```python
from build123d import *

# Parameters (mm, degrees)
F0_W     = 75
F0_H     = 21.8987613916
F1_DEPTH = 14
F3_DEPTH = 21.8997613916
F4_W     = 23.978275167
F4_H     = 7.947247941
F4_W_2   = 48.6262406095
F5_DEPTH = 25
F6_W     = 7.6308213174
F6_H     = 13.8987613916
F6_W_2   = 6.0403123498
F6_W_3   = 10.3618325666
F7_DEPTH = 6


with BuildPart() as f1:
    # F0 (on Top) → F1 (new body)
    with BuildSketch(Plane.XY):
        with Locations((37.5, 10.9493806958)):
            Rectangle(F0_W, F0_H)
    extrude(amount=F1_DEPTH)

    # F2 (on face) → F3 (cut, through all)
    with BuildSketch(Plane.XZ):
        Polygon((0, 14), (0, 6.3767037354), (5.3324829787, 14), align=None)
        Polygon((68.8854381442, 14), (11.3727953285, 14), (13.736397028, 6.2453923747), (62.3593553901, 6.8103666529), (63.1077513099, 9.8052984104), (65.2087256312, 11.3810319453), (67.0470818877, 12.6941427588), align=None)
        Polygon((75, 14), (70.9864199162, 14), (73.8660361752, 12.6941427588), (75, 10.330542922), align=None)
        Polygon((67.3934295774, 4.770135507), (67.3934295774, 0), (75, 0), (75, 2.5454831775), (74.345, 2.5454831775), (74.345, 4.770135507), align=None)
        Polygon((2.3223445751, 6.9947880693), (0, 4.561574664), (0, 0), (9.3439053744, 2.0588401239), (8.8216059457, 6.9350752235), (8.1620588899, 7.2728698142), (6.6326097585, 4.2866062695), (5.1598150908, 4.2866062695), align=None)
    extrude(amount=-F3_DEPTH, mode=Mode.SUBTRACT)

    # F4 (on face) → F5 (cut)
    with BuildSketch(Plane(origin=(-0.0707041789, 0, 6.0849608152), x_dir=(0.9999325005, 0, 0.0116187119), z_dir=(-0.0116187119, 0, 0.9999325005))):
        with Locations((74.4234114354, 11.0779821407)):
            Rectangle(F4_W, F4_H)
        with Locations((38.1211535471, 11.0779821407)):
            Rectangle(F4_W_2, F4_H)
    extrude(amount=F5_DEPTH, mode=Mode.SUBTRACT)

    # F6 (on face) → F7 (cut)
    with BuildSketch(Plane.XY.offset(14)):
        with Locations((15.1882059872, 10.9493806958)):
            Rectangle(F6_W, F6_H)
        with Locations((8.3526391536, 10.9493806958)):
            Rectangle(F6_W_2, F6_H)
        with Locations((0.1515666954, 10.9493806958)):
            Rectangle(F6_W_3, F6_H)
    extrude(amount=-F7_DEPTH, mode=Mode.SUBTRACT)


solid = f1.part
```
Source: CAD feature listing. Evaluate the final solid. Frame: model axes, mm. A direction names the side the tool comes from. Give positions to 0.01 mm unless a question says otherwise; leave off trailing zeros. Order: outer loops, then holes, each group sorted by start corner. A loop starts at its lowest first (then second) coordinate and runs counter-clockwise, first axis right, second up.
(1) Section query C-C (x = 19). Return the cut outline in (y, z), plus the area to 3 significant figures.
(2) Contact query for flat-ended pins moving along their axis: P1, Ø5, axis at x = 27.5, y = 9.5, coming from the -Z side; P2, Ø0.7, axis at y = 15.5, z = 3.5, coming from the -X side; P3, Ø0.7, axis at x = 75, y = 7, coming from the -Z side; P4, Ø8, axis at x = 44, y = 15.5, coming from the +Z side. Output: stop coordinate, or through.
(3) Access query for faces 1 (the face through (4.607, 10.796, 1.015)), 2 (the face through (1.18, 10.8, 5.8)), 3 (the face through (64.14, 18.43, 10.58)). Directions: +Z, -Z, +X, -X, +Y, -Y. A direction counts if a zero-diameter tool reaches every point of the face in a straight line with its end or side. Return the directions, or none.
(4) Section query A-A (y = 20). Return the cut outline in (x, z) (3 decimals), plus the area to 3 significant figures.
(5) Material intervals for line 1 along Y through (x, z) = (64, 10); line 2 along Y through (x, z) = (8, 13); line 3 along X through (y, z) = (5, 4) (3 decimals), sorted ascending.
(6) Pull-direction query (X, two-part tool) for faces 4 (the face through (67.953, 18.427, 13.338)), 5 (the face through (0, 11, 5)), 6 (the face through (33, 11, 0)); classes: +X half, -X half, draft (parallel to the pull), parting line (faces both ways), or undercut.
(7) Section query D-D (x = 61). Return the cut outline in (y, z), plus the area to 3 significant figures.
(8) Section query B-B (y = 5.25). Return the cut outline in (x, z) (1 decimal), plus the area to 3 significant figures.
Outcome:
1. outline: (0, 0) - (21.9, 0) - (21.9, 6.31) - (0, 6.31) - close
1. area: 138 mm2
2. P1: stops at z = 0
2. P2: stops at x = 9.15
2. P3: stops at z = 2.55
2. P4: stops at z = 6.64
3. face 1: -X, +Y, -Y
3. face 2: +Y, -Y
3. face 3: +Z, +Y, -Y
4. outline: (0, 0) - (67.393, 0) - (67.393, 4.77) - (74.345, 4.77) - (74.345, 2.545) - (75, 2.545) - (75, 10.331) - (73.866, 12.694) - (70.986, 14) - (68.885, 14) - (67.047, 12.694) - (65.209, 11.381) - (63.108, 9.805) - (62.359, 6.81) - (13.736, 6.245) - (11.373, 14) - (5.332, 14) - (0, 6.377) - (0, 4.562) - (2.322, 6.995) - (5.16, 4.287) - (6.633, 4.287) - (8.162, 7.273) - (8.822, 6.935) - (9.344, 2.059) - close
4. area: 559 mm2
5. line 1: y = 0 to 7.1, 15.05 to 21.9
5. line 2: y = 0 to 4, 17.9 to 21.9
5. line 3: x = 9.136 to 67.393, 74.345 to 75
6. face 4: undercut
6. face 5: -X half
6. face 6: draft
7. outline: (0, 0) - (21.9, 0) - (21.9, 6.79) - (0, 6.79) - close
7. area: 149 mm2
8. outline: (0, 0) - (67.4, 0) - (67.4, 4.8) - (74.3, 4.8) - (74.3, 2.5) - (75, 2.5) - (75, 10.3) - (73.9, 12.7) - (71, 14) - (68.9, 14) - (67, 12.7) - (65.2, 11.4) - (63.1, 9.8) - (62.4, 6.8) - (13.7, 6.2) - (13.2, 8) - (1.1, 8) - (0, 6.4) - (0, 4.6) - (2.3, 7) - (5.2, 4.3) - (6.6, 4.3) - (8.2, 7.3) - (8.8, 6.9) - (9.3, 2.1) - close
8. area: 505 mm2
